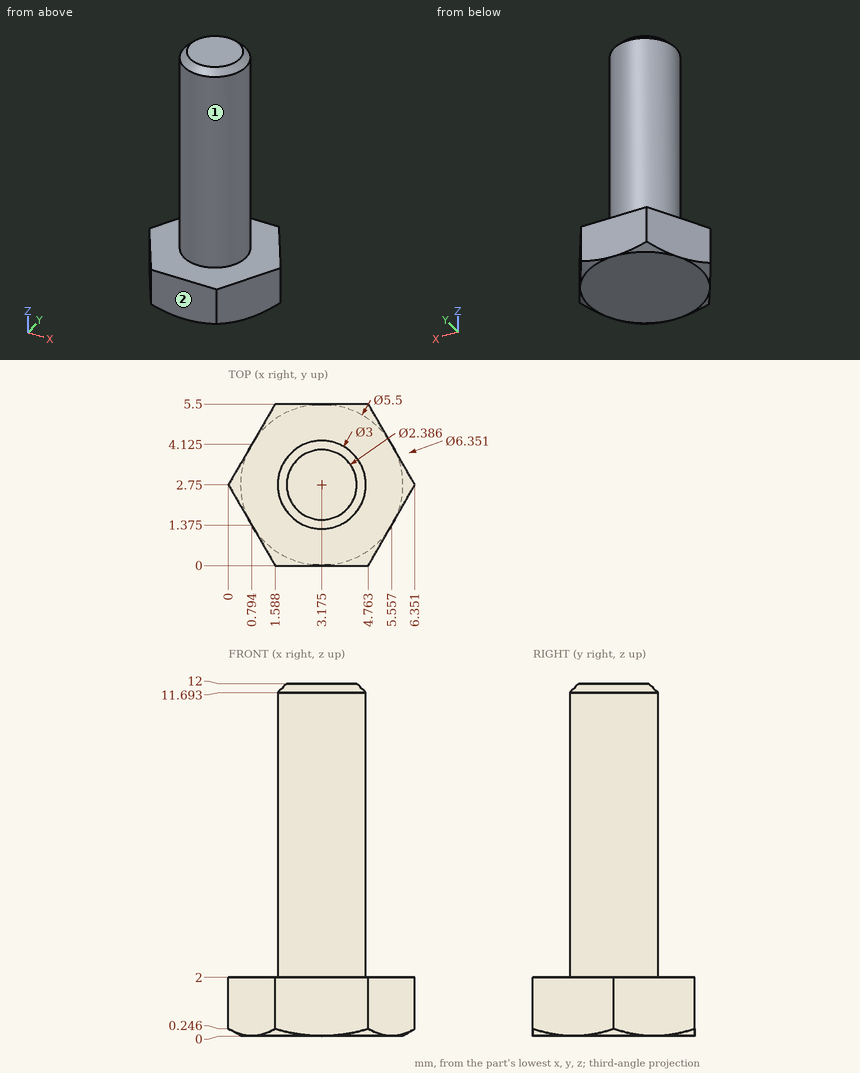
Study the drawing (mm; zero at the part's minimum x, y, z) and answer. A direction names the side the tool comes from. Coordinates: 2 decimals unless noted, no trailing zeros. Answer in a Markdown table with one row per item. Add a question column.
1. Consider L1, parallel to X at y = 2.7, z = 7.5 (1 decimal); L2, parallel to Z at x = 5, y = 3.15; L3, parallel to X at y = 3.95, z = 11.25 (1 decimal). Determine where each line is inside the solid, lowest interval first.
2. A flat-ended cylindrical pin translates along its axis: P1, Ø2, axis at x = 1.5, z = 8.5, coming from the -Y side. Find the tip coordinate at first contact, or state that the pin passes through.
3. A tool of negligible diameter and unlimited length cuts with its end or side. For the marked faces 1 and 2, from which of +Z, -Z, +X, -X, +Y, -Y can it reach the whole face along a straight path? Write none if from no direction.
Reported:
| question | item | result |
|---|---|---|
| 1 | L1 | x = 1.7 to 4.7 |
| 1 | L2 | z = 0 to 2 |
| 1 | L3 | x = 2.3 to 4.1 |
| 2 | P1 | stops at y = 1.41 |
| 3 | face 1 | +Z |
| 3 | face 2 | +Z, -Z, +X, -X, -Y |
